```python
from build123d import *

# Parameters (mm, degrees)
CYLINDER_R           = 2.95
CYLINDER_DEPTH       = 7
CYLINDER001_R        = 1.7
CYLINDER001_DEPTH    = 30
CLONE062_PITCH_ANGLE = -90
CLONE061_PITCH_ANGLE = -90
BOX246_W             = 10
BOX246_H             = 6.9
BOX246_DEPTH         = 34
CYLINDER1003_R       = 8.2
CYLINDER1003_DEPTH   = 15
CLONE058_PITCH_ANGLE = 90


with BuildPart() as m3bolthead:
    # Cylinder → Cylinder (new body)
    with BuildSketch(Plane.XY):
        Circle(CYLINDER_R)
    extrude(amount=CYLINDER_DEPTH)


with BuildPart() as m3bolt:
    # Cylinder001 → Cylinder001 (new body)
    with BuildSketch(Plane.XY.offset(6)):
        Circle(CYLINDER001_R)
    extrude(amount=CYLINDER001_DEPTH)

    # Fusion: union M3BoltHead
    add(m3bolthead.part)


with BuildPart() as clone_of_m3bolt022:
    # Clone062 base: copy of M3Bolt
    add(m3bolt.part)


with BuildPart() as clone_of_m3bolt022_1:
    # Clone062 pitch: moved
    add(clone_of_m3bolt022.part.rotate(Axis((0, 0, 0), (0, 1, 0)), CLONE062_PITCH_ANGLE))


with BuildPart() as clone_of_m3bolt022_2:
    # Clone062 placement: moved
    add(clone_of_m3bolt022_1.part.moved(Location((36, 0, -11))))


with BuildPart() as clone_of_m3bolt021:
    # Clone061 base: copy of M3Bolt
    add(m3bolt.part)


with BuildPart() as clone_of_m3bolt021_1:
    # Clone061 pitch: moved
    add(clone_of_m3bolt021.part.rotate(Axis((0, 0, 0), (0, 1, 0)), CLONE061_PITCH_ANGLE))


with BuildPart() as clone_of_m3bolt021_2:
    # Clone061 placement: moved
    add(clone_of_m3bolt021_1.part.moved(Location((36, 0, 11))))


with BuildPart() as cube010:
    # Box246 → Box246 (new body)
    with BuildSketch(Plane(origin=(2, -3.45, -17), x_dir=(1, 0, 0), z_dir=(0, 0, 1))):
        with Locations((5, 3.45)):
            Rectangle(BOX246_W, BOX246_H)
    extrude(amount=BOX246_DEPTH)


with BuildPart() as fusion021:
    # Cylinder1003 → Cylinder1003 (new body)
    with BuildSketch(Plane.XY):
        Circle(CYLINDER1003_R)
    extrude(amount=CYLINDER1003_DEPTH)


with BuildPart() as fusion021_1:
    # Clone058 pitch: moved
    add(fusion021.part.rotate(Axis((0, 0, 0), (0, 1, 0)), CLONE058_PITCH_ANGLE))


with BuildPart() as fusion021_2:
    # Clone058 placement: moved
    add(fusion021_1.part)

    # Fusion021: union Clone of M3Bolt022, Clone of M3Bolt021, Cube010
    add(clone_of_m3bolt022_2.part)
    add(clone_of_m3bolt021_2.part)
    add(cube010.part)


with BuildPart() as obj1:
    # Sketch016 → Revolution003 (revolve)
    with BuildSketch(Plane.XY):
        Polygon((0, 0), (0, 18), (6, 12), (6, 0), align=None)
    revolve(axis=Axis((0, 0, 0), (1, 0, 0)))

    # Cut020: cut Fusion021
    add(fusion021_2.part, mode=Mode.SUBTRACT)


solid = obj1.part
```
Build history of the part. All positions in model axes, mm. A direction names the side the tool comes from. Round coordinates to 2 decimals unless told otherwise and drop trailing zeros. Write each loop counter-clockwise with the first axis right and the second up, starting at its lowest first coordinate (ties: lowest second). Pieces come first, ordered by that corner, then holes. Notation, with made-up numbers: (-37.75, 67.5) - (-27.75, 67.5) arc R29 cw to (-27.75, 102.5) - close; hole circle Ø10 at (-6.75, -35). An arc over 180 degrees is marked (long way). Write each question's results on one line, items separated by ' | '. Start each with the question number.
Item 1: Drop flat-ended pins along their axis: P1, Ø1, axis at x = 3, z = -9.5, coming from the +Y side; P2, Ø3.5, axis at y = -1.5, z = 11, coming from the +X side; P3, Ø2.5, axis at y = 0, z = -11, coming from the -X side; P4, Ø3, axis at x = 5, z = -4.5, coming from the +Y side. Give the stop position or say it passes through.
Item 2: Mould opens along Z. For faces 3 (the face through (4, -3.45, -11)), 4 (the face through (1.01, -0.65, -9.43)), 5 (the face through (5.709, 11.724, 3.692)) say: pulls with the +Z half, pulls with the -Z half, needs draft (parallel to the pull), parting line crosses it, or undercut.
Item 3: Which spindle directions (+Z, -Z, +X, -X, +Y, -Y) get a long thin tool onto all of the face, cutting with end or side? Do faces 1 (the face through (2, -1, 13)), 2 (the face through (1.01, -1.66, 10.63)). Say none if no direction does.
Item 4: Saw through at B-B (z = 0). Write the cut outline in (x, y).
Item 5: Saw through at C-C (x = 1.25). Write the cut outline in (y, z), and give its area (3 significant figures).
Item 6: Wall check: L1, parallel to Y at x = 1, z = -9.5; L2, parallel to X at y = -1, z = -9; L3, parallel to Z at x = 0.95, y = 0. Give the ranges that are in metal, low to high. Write a range as [from, to].
Item 7: Saw through at A-A (y = 0). Write the cut outline in (x, z), and give its area (3 significant figures).
Results are:
1) P1: stops at y = 12.35 | P2: stops at x = 2 | P3: passes through | P4: stops at y = 13.85
2) face 3: needs draft | face 4: undercut | face 5: parting line crosses it
3) face 1: +Z, -Z, +X | face 2: +X, -X
4) outline: (0, -18) - (6, -12) - (6, -8.2) - (0, -8.2) - close; (0, 8.2) - (6, 8.2) - (6, 12) - (0, 18) - close
5) outline: circle Ø33.5 at (0, 0); hole circle Ø16.4 at (0, 0); hole circle Ø3.4 at (0, -11); hole circle Ø3.4 at (0, 11) | area: 652 mm²
6) L1: y = [-14.1, -0.8], [0.8, 14.1] | L2: x = [0, 2] | L3: z = [-17.05, -12.7], [-9.3, -8.2], [8.2, 9.3], [12.7, 17.05]
7) outline: (0, -18) - (2, -16) - (2, -12.7) - (0, -12.7) - close; (0, -9.3) - (2, -9.3) - (2, -8.2) - (0, -8.2) - close; (0, 8.2) - (2, 8.2) - (2, 9.3) - (0, 9.3) - close; (0, 12.7) - (2, 12.7) - (2, 16) - (0, 18) - close | area: 21.6 mm²
